CAD build for the part. Positions are in the model's coordinates, mm. Face numbers are marked on the shaded views. A direction names the side the tool comes from. Round coordinates to 2 decimals unless told otherwise and drop trailing zeros. Write each loop counter-clockwise with the first axis right and the second up, starting at its lowest first coordinate (ties: lowest second). Pieces come first, ordered by that corner, then holes. Notation, with made-up numbers: (82, 37) - (94, 37) arc R21 cw to (94, 42) - close; hole circle Ø10 at (-15, 65). An arc over 180 degrees is marked (long way). Put each result on its own line as item: value. Start each with the question number.
Item 1: Cut at D-D (y = 7.75). Give the cut face in (x, z), and give its area (3 significant figures).
Item 2: 3-axis set-ups, long thin cutter, end or side, ignore diameter. For the marked faces 5, 6, 7, 8 and 9: which of +Z, -Z, +X, -X, +Y, -Y reach the whole face in a straight line?
Item 3: Mould opens along X. For the marked faces 1, 2, 3 and 4 say: released by +X, released by -X, zero draft, split by the parting line, or undercut.
Item 4: Drill centre lines: line 1 (Y direction, x = 0, z = 12.75); line 2 (X direction, y = 1.25, z = 22); line 3 (X direction, y = 1.75, z = 11.5). Where is each one in solid material? Low to high. Write a range as from..to.
Item 5: Cut at B-B (z = 13.5). Give the cut face in (x, y).
Item 6: Cut at A-A (x = 0). Give the cut face in (y, z) (3 decimals).
Item 7: Pin check, flat tips, straight feed: pin 1 Ø0.7 at (x, z) = (0.5, 2) entering from +Y (3 decimals); pin 2 Ø2.5 at (y, z) = (0.5, 2) entering from -X (3 decimals); pin 3 Ø4 at (x, z) = (1, 1.5) entering from -Y (3 decimals). Stop position of each tip, or through.
Item 8: Cut at C-C (y = 5.75). Give the cut face in (x, z), and give its area (3 significant figures).
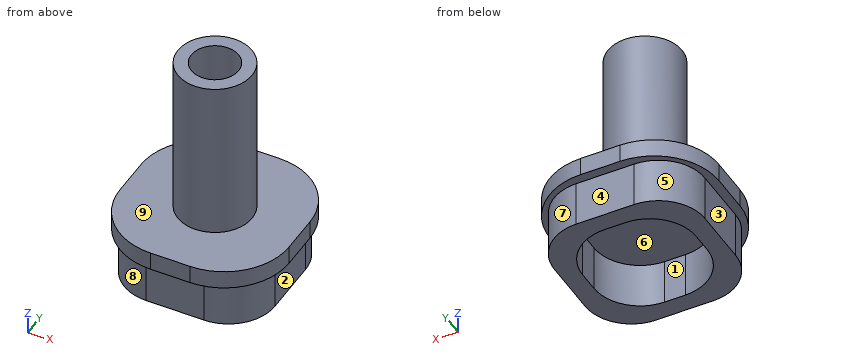
```python
from build123d import *

# Parameters (mm, degrees)
SKETCH1_W           = 16.25
SKETCH1_H           = 16.25
SKETCH1_W_2         = 12.25
SKETCH1_H_2         = 12.25
BOSS_EXTRUDE1_DEPTH = 5
FILLET1_R           = 5
SKETCH2_W           = 18.25
SKETCH2_H           = 18.25
BOSS_EXTRUDE2_DEPTH = 2
FILLET2_R           = 7
SKETCH4_R           = 4
BOSS_EXTRUDE3_DEPTH = 17.7
SKETCH6_R           = 2.55
CUT_EXTRUDE1_DEPTH  = 16.7


with BuildPart() as part:
    # Sketch1 → Boss-Extrude1 (new body)
    with BuildSketch(Plane.XY):
        Rectangle(SKETCH1_W, SKETCH1_H)
        Rectangle(SKETCH1_W_2, SKETCH1_H_2, mode=Mode.SUBTRACT)
    extrude(amount=BOSS_EXTRUDE1_DEPTH)

    # Fillet1
    fillet1_edges = [part.edges().sort_by_distance(p)[0] for p in [
        (6.125, -6.125, 2.5),
        (6.125, 6.125, 2.5),
        (-6.125, 6.125, 2.5),
        (-6.125, -6.125, 2.5),
        (-8.125, 8.125, 2.5),
        (8.125, 8.125, 2.5),
        (8.125, -8.125, 2.5),
        (-8.125, -8.125, 2.5),
    ]]
    fillet(fillet1_edges, radius=FILLET1_R)

    # Sketch2 → Boss-Extrude2 (add)
    with BuildSketch(Plane.XY.offset(5)):
        Rectangle(SKETCH2_W, SKETCH2_H)
    extrude(amount=BOSS_EXTRUDE2_DEPTH)

    # Fillet2
    fillet2_edges = [part.edges().sort_by_distance(p)[0] for p in [
        (-9.125, 9.125, 6),
        (-9.125, -9.125, 6),
        (9.125, -9.125, 6),
        (9.125, 9.125, 6),
    ]]
    fillet(fillet2_edges, radius=FILLET2_R)

    # Sketch4 → Boss-Extrude3 (add)
    with BuildSketch(Plane.XY.offset(7)):
        Circle(SKETCH4_R)
    extrude(amount=BOSS_EXTRUDE3_DEPTH)

    # Sketch6 → Cut-Extrude1 (cut)
    with BuildSketch(Plane.XY.offset(24.7)):
        Circle(SKETCH6_R)
    extrude(amount=-CUT_EXTRUDE1_DEPTH, mode=Mode.SUBTRACT)


solid = part.part
```
Output values:
1. outline: (-6.29, 5) - (-5.02, 5) - (-5.02, 0) - (5.02, 0) - (5.02, 5) - (6.29, 5) - (6.29, 7) - (-6.29, 7) - close
1. area: 75.4 mm2
2. face 5: -Z, -X, +Y
2. face 6: -Z
2. face 7: -Z, +X, +Y
2. face 8: -Z, -X, -Y
2. face 9: +Z
3. face 1: undercut
3. face 2: released by +X
3. face 3: released by -X
3. face 4: zero draft
4. line 1: -4..-2.55, 2.55..4
4. line 2: -3.8..-2.22, 2.22..3.8
4. line 3: -3.6..-1.85, 1.85..3.6
5. outline: circle Ø8 at (0, 0); hole circle Ø5.1 at (0, 0)
6. outline: (-9.125, 5) - (-8.125, 5) - (-8.125, 0) - (-6.125, 0) - (-6.125, 5) - (6.125, 5) - (6.125, 0) - (8.125, 0) - (8.125, 5) - (9.125, 5) - (9.125, 7) - (4, 7) - (4, 24.7) - (2.55, 24.7) - (2.55, 8) - (-2.55, 8) - (-2.55, 24.7) - (-4, 24.7) - (-4, 7) - (-9.125, 7) - close
7. pin 1: y = 8.125
7. pin 2: x = -8.125
7. pin 3: y = -8.125
8. outline: (-8.11, 5) - (-7.38, 5) - (-7.38, 0) - (-3.02, 0) - (-3.02, 5) - (3.02, 5) - (3.02, 0) - (7.38, 0) - (7.38, 5) - (8.11, 5) - (8.11, 7) - (-8.11, 7) - close
8. area: 76.0 mm2
